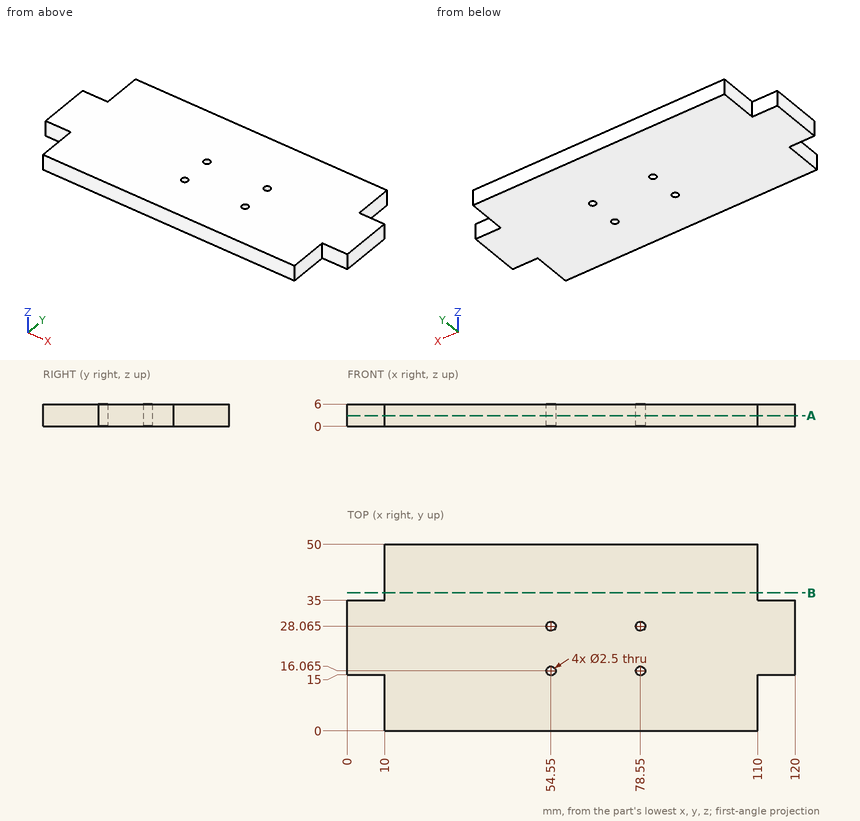
Could you check a few things on this drawing? It's one solid part, dimensions in mm from its lowest x, y, z. Give positions to 0.01 mm unless a question says otherwise; leave off trailing zeros. Write each loop counter-clockwise with the first axis right and the second up, starting at its lowest first coordinate (ties: lowest second). Pieces come first, ordered by that corner, then holes.
(1) Imagine slicing it at B-B, the plane y = 37. Write out the boundary of the cut face in (x, z), and give its area (3 significant figures).
Output values:
outline: (10, 0) - (110, 0) - (110, 6) - (10, 6) - close
area: 600 mm2
(2) Imagine slicing it at A-A, the plane z = 2.9. Count the separate pieces of the cut face and the enclosed holes in it, and give its area (3 significant figures).
Output values:
separate pieces: 1
enclosed holes: 4
area: 5,380 mm2
(3) If I drill on L1, parallel to X at y = 28.5, z = 5.6; L2, parallel to X at y = 6, z = 1.75; L3, parallel to Y at x = 6, z = 3.9, over which ranges is the centre line in solid material (lowest first)?
Output values:
L1: x = 0 to 53.38, 55.72 to 77.38, 79.72 to 120
L2: x = 10 to 110
L3: y = 15 to 35
(4) Will these pins go through, and if not, where does the flat tip stop? pin 1 (1.5 mm diameter, centred on y = 9.5, z = 5, fed in from +X); pin 2 (3 mm diameter, centred on x = 7, z = 2.5, fed in from +Y); pin 3 (2 mm diameter, centred on y = 45, z = 1.5, fed in from -X).
Output values:
pin 1: stops at x = 110
pin 2: stops at y = 35
pin 3: stops at x = 10
